Input: part model. Units: mm. Frame: model coordinates. Coordinates: 2 decimals unless noted, no trailing zeros. Loops run counter-clockwise (first coordinate to the right, second up) from the corner with the lowest first, then second, coordinate; pieces in that order, holes last.
```python
from build123d import *

# Parameters (mm, degrees)
SKETCH_R                  = 1.65
PAD_DEPTH                 = 10
SKETCH001_W               = 140.265109
SKETCH001_H               = 100
PAD003_DEPTH              = 5
FUSION008_PLACEMENT_ANGLE = 180


with BuildPart() as pad:
    # Sketch → Pad (new body)
    with BuildSketch(Plane.XY):
        with Locations((4.180322, -22.326468)):
            Circle(SKETCH_R)
        with Locations((4.180322, 28.473532)):
            Circle(SKETCH_R)
        with Locations((54.980322, -17.226468)):
            Circle(SKETCH_R)
        with Locations((54.980322, 10.673532)):
            Circle(SKETCH_R)
    extrude(amount=PAD_DEPTH)


with BuildPart() as cut:
    # Sketch001 → Pad003 (new body)
    with BuildSketch(Plane.XY):
        with Locations((54.553008, 0)):
            Rectangle(SKETCH001_W, SKETCH001_H)
    extrude(amount=PAD003_DEPTH)

    # Cut: cut Pad
    add(pad.part, mode=Mode.SUBTRACT)


with BuildPart() as placa:
    # Cone → Cone (revolve)
    with BuildSketch(Plane(origin=(109, 0, 0), x_dir=(1, 0, 0), z_dir=(0, -1, 0))):
        Polygon((0, 0), (10, 0), (4, 30), (0, 30), align=None)
    revolve(axis=Axis((109, 0, 0), (0, 0, 1)))

    # Fusion008: union Cut
    add(cut.part)


with BuildPart() as placa_1:
    # Fusion008 placement: moved
    add(placa.part.moved(Location((109, 0, 30))).rotate(Axis((109, 0, 30), (0, 1, 0)), FUSION008_PLACEMENT_ANGLE))


solid = placa_1.part
```
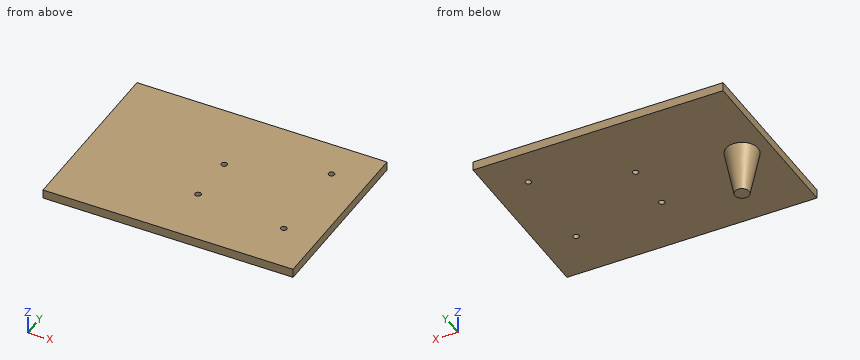
Item 1: Section query B-B (x = 0). Output: boundary loops of the cut face in (y, z).
Result:
outline: (-50, 25) - (-9, 25) - (-4, 0) - (4, 0) - (9, 25) - (50, 25) - (50, 30) - (-50, 30) - close
Item 2: Contact query for flat-ended pins moving along their axis: P1, Ø2, axis at x = 16, y = 7.5, coming from the -Z side; P2, Ø1, axis at y = -1, z = 16, coming from the +X side. Output: stop coordinate, or through.
Result:
P1: stops at z = 25
P2: stops at x = 7.25
Item 3: Section query D-D (x = 22). Output: boundary loops of the cut face in (y, z), then the cut area to 3 significant figures.
Result:
outline: (-50, 25) - (50, 25) - (50, 30) - (-50, 30) - close
area: 500 mm2
Item 4: Section query C-C (z = 3). Output: boundary loops of the cut face in (x, y).
Result:
outline: circle Ø9.2 at (0, 0)
Item 5: Line query: L1, parallel to Z at x = 21.5, y = -40.5; L2, parallel to Y at x = -5, z = 8. Output: solid intervals per line, ascending.
Result:
L1: z = 25 to 30
L2: y = -2.52 to 2.52
Item 6: Section query A-A (y = 0). Output: boundary loops of the cut face in (x, z), then the cut area to 3 significant figures.
Result:
outline: (-15.69, 25) - (-9, 25) - (-4, 0) - (4, 0) - (9, 25) - (124.58, 25) - (124.58, 30) - (-15.69, 30) - close
area: 1,030 mm2
